```python
from build123d import *

# Parameters (mm, degrees)
SKETCH2_W           = 76.2
SKETCH2_H           = 25.4
SKETCH2_R           = 2.5
BOSS_EXTRUDE1_DEPTH = 6.35
SKETCH3_W           = 25.4
SKETCH3_H           = 190.5
BOSS_EXTRUDE2_DEPTH = 6.35
BOSS_EXTRUDE3_DEPTH = 5.08
SKETCH5_R           = 7.5
CUT_EXTRUDE1_DEPTH  = 37.592


with BuildPart() as part:
    # Sketch2 → Boss-Extrude1 (new body)
    with BuildSketch(Plane(origin=(0, 0, 0), x_dir=(1, 0, 0), z_dir=(0, 1, 0))):
        Rectangle(SKETCH2_W, SKETCH2_H)
        with Locations((-25.4, 0)):
            Circle(SKETCH2_R, mode=Mode.SUBTRACT)
        with Locations((25.4, 0)):
            Circle(SKETCH2_R, mode=Mode.SUBTRACT)
    extrude(amount=BOSS_EXTRUDE1_DEPTH)

    # Sketch3 → Boss-Extrude2 (add)
    with BuildSketch(Plane(origin=(38.1, 0, 0), x_dir=(0, 0, -1), z_dir=(1, 0, 0))):
        with Locations((0, 95.25)):
            Rectangle(SKETCH3_W, SKETCH3_H)
    extrude(amount=BOSS_EXTRUDE2_DEPTH)


with BuildPart() as body_2:
    # Sketch4 → Boss-Extrude3 (new body)
    with BuildSketch(Plane.XY.offset(12.7)):
        Polygon((22.9, 6.35), (27.9, 6.35), (38.1, 6.35), (38.1, 98.425), (0, 6.35), align=None)
    extrude(amount=-BOSS_EXTRUDE3_DEPTH)


with BuildPart() as body_3:
    # Mirror2: mirrored copy
    add(body_2.part.mirror(Plane.XY))


with BuildPart() as body_2_1:
    add(body_2.part)

    # Combine1: union body 3, part
    add(body_3.part)
    add(part.part)

    # Sketch5 → Cut-Extrude1 (cut)
    with BuildSketch(Plane(origin=(44.45, 0, 0), x_dir=(0, 0, -1), z_dir=(1, 0, 0))):
        with Locations((0, 190.5)):
            Circle(SKETCH5_R)
    extrude(amount=-CUT_EXTRUDE1_DEPTH, mode=Mode.SUBTRACT)


solid = body_2_1.part
```
Source: CAD feature listing. Evaluate the final solid. Frame: model axes, mm. A direction names the side the tool comes from. Round coordinates to 2 decimals unless told otherwise and drop trailing zeros. Loops run counter-clockwise (first coordinate to the right, second up) from the corner with the lowest first, then second, coordinate; pieces in that order, holes last. Notation, with made-up numbers: M -24,26 L 28,26 A16 cw 28,38 Z; hole C 76,41.5 d9. An arc over 180 degrees is marked long. Use a Markdown table: item, result. Add a question column.
1. Mould query, pull axis X, two halves, no side actions, for faces 1 (the flat face through (44.45, 97, 0)), 2 (the cylindrical face through (27.71, 3.13, 0.96)), 3 (the flat face through (27, 33, 7.62)). Classes: pulls with the +X half, pulls with the -X half, needs draft (parallel to the pull), parting line crosses it, or undercut.
2. Section query D-D on x = 36. Return the cut outline in (y, z).
3. Line query: line 1 (X direction, y = 1.5, z = 0); line 2 (Z direction, x = 25, y = 5); line 3 (Y direction, x = 26.5, z = 5.25). Output: solid intervals per line, ascending.
4. Contact query for flat-ended pins moving along their axis: P1, Ø4, axis at x = 25.4, z = 0, coming from the +Y side; P2, Ø6, axis at y = 146.5, z = 1.5, coming from the -X side. Output: stop coordinate, or through.
5. Section query C-C on y = 90.5. Return the cut outline in (x, z).
6. Reachability of faces 4 (the flat face through (24, 52, 12.7)), 5 (the flat face through (38.1, 120, 0)) from +Z, -Z, +X, -X, +Y, -Y: full face, straight path, thin tool, end or side. Return the list, or none.
7. Section query B-B on z = 0. Return the cut outline in (x, y), then the cut area to 3 significant figures.
8. Section query A-A on x = -25.4. Return the cut outline in (y, z), then the cut area to 3 significant figures.
Reported:
| question | item | result |
|---|---|---|
| 1 | face 1 | pulls with the +X half |
| 1 | face 2 | undercut |
| 1 | face 3 | needs draft |
| 2 | outline | M 0,-12.7 L 93.35,-12.7 L 93.35,-7.62 L 6.35,-7.62 L 6.35,7.62 L 93.35,7.62 L 93.35,12.7 L 0,12.7 Z |
| 3 | line 1 | x = -38.1 to -27.9, -22.9 to 22.9, 27.9 to 44.45 |
| 3 | line 2 | z = -12.7 to -2.47, 2.47 to 12.7 |
| 3 | line 3 | y = 0 to 6.35 |
| 4 | P1 | passes through |
| 4 | P2 | stops at x = 38.1 |
| 5 | outline | M 34.82,-12.7 L 44.45,-12.7 L 44.45,12.7 L 34.82,12.7 L 34.82,7.62 L 38.1,7.62 L 38.1,-7.62 L 34.82,-7.62 Z |
| 6 | face 4 | +Z, +X, -X, +Y, -Y |
| 6 | face 5 | -X, +Y |
| 7 | outline | M -38.1,0 L -27.9,0 L -27.9,6.35 L -38.1,6.35 Z; M -22.9,0 L 22.9,0 L 22.9,6.35 L -22.9,6.35 Z; M 27.9,0 L 44.45,0 L 44.45,183 L 38.1,183 L 38.1,6.35 L 27.9,6.35 Z |
| 7 | area | 1,580 mm² |
| 8 | outline | M 0,-12.7 L 6.35,-12.7 L 6.35,-2.5 L 0,-2.5 Z; M 0,2.5 L 6.35,2.5 L 6.35,12.7 L 0,12.7 Z |
| 8 | area | 130 mm² |
